from build123d import *

# Parameters (mm, degrees)
F0_W     = 25.4
F0_H     = 25.4
F1_DEPTH = 50.8
F2_W     = 20.32
F2_H     = 45.72
F3_DEPTH = 22.86
F4_R     = 3.175
F4_R_2   = 1.905
F5_DEPTH = 10.16
F6_DEPTH = 25.4
F7_R     = 5.08
F8_DEPTH = 2.54


with BuildPart() as f1:
    # F0 (on Top) → F1 (new body)
    with BuildSketch(Plane.XY):
        with Locations((-10.5220779449, -6.5101005034)):
            Rectangle(F0_W, F0_H)
    extrude(amount=F1_DEPTH)

    # F2 (on face) → F3 (cut)
    with BuildSketch(Plane(origin=(0, 6.1898994966, 0), x_dir=(-1, 0, 0), z_dir=(0, 1, 0))):
        with Locations((10.5220779449, 25.4)):
            Rectangle(F2_W, F2_H)
    extrude(amount=-F3_DEPTH, mode=Mode.SUBTRACT)

    # F4 (on face) → F5 (join)
    with BuildSketch(Plane(origin=(0, -16.6701005034, 0), x_dir=(-1, 0, 0), z_dir=(0, 1, 0))):
        with Locations((11.9491452351, 36.013584584)):
            Circle(F4_R)
        with Locations((11.9491452351, 36.013584584)):
            Circle(F4_R_2, mode=Mode.SUBTRACT)
        with Locations((11.369979009, 16.9800035655)):
            Circle(F4_R)
        with Locations((11.369979009, 16.9800035655)):
            Circle(F4_R_2, mode=Mode.SUBTRACT)
    extrude(amount=F5_DEPTH)

    # F6 (cut): faces of the model
    f6_faces = [f1.faces().sort_by_distance(p)[0] for p in [
        (-11.9491452351, -16.6701005034, 36.013584584),
        (-11.369979009, -16.6701005034, 16.9800035655),
    ]]
    extrude(f6_faces, amount=-F6_DEPTH, mode=Mode.SUBTRACT)

    # F7 (on face) → F8 (join)
    with BuildSketch(Plane(origin=(0, -16.6701005034, 0), x_dir=(-1, 0, 0), z_dir=(0, 1, 0))):
        with Locations((11.369979009, 16.9800035655)):
            Circle(F7_R)
        with Locations((11.9491452351, 36.013584584)):
            Circle(F7_R)
    extrude(amount=F8_DEPTH)


solid = f1.part
Build history of the part. All positions in model axes, mm. A direction names the side the tool comes from. Give positions to 0.01 mm unless a question says otherwise; leave off trailing zeros. Write each loop counter-clockwise with the first axis right and the second up, starting at its lowest first coordinate (ties: lowest second). Pieces come first, ordered by that corner, then holes. Notation, with made-up numbers: (75, -18.75) - (101, -18.75) arc R31 ccw to (101, 15.25) - close; hole circle Ø4 at (33.5, -35.75). An arc over 180 degrees is marked (long way). Use one line per item in the form item = value. Start each with the question number.
1. Band-saw the part on B-B on y = 4. Write the cut outline in (x, z).
2. Band-saw the part on C-C on z = 4. Write the cut outline in (x, y).
3. Band-saw the part on A-A on y = -12. Write the cut outline in (x, z) (3 decimals).
4. Band-saw the part on D-D on x = -18.5. Write the cut outline in (y, z).
5. Drop flat-ended pins along their axis: pin 1 Ø3 at (x, z) = (-11.95, 36.01) entering from +Y; pin 2 Ø8 at (x, z) = (-12, 33.5) entering from +Y; pin 3 Ø5 at (x, z) = (-3.5, 28.5) entering from +Y. Give the stop position or say it passes through.
6. Probe line 1 (Z direction, x = -17.5, y = -13.5); line 2 (X direction, y = -4, z = 32); line 3 (Z direction, x = -12.5, y = -10.5). List the from-to ranges inside material, lowest first. Write a range as [from, to].
7. Two-plate mould, pull along Z, no slides. Class faces 4 (the face through (-23.222, -7, 25)), 5 (the face through (-11, -6, 0)), 6 (the face through (-10, -5, 48.26)): released by +Z, released by -Z, zero draft, split by the parting line, or undercut.
8. 3-axis set-ups, long thin cutter, end or side, ignore diameter. For faces 1 (the face through (-11, -6, 50.8)), 2 (the face through (-12.25, -10.37, 15.29)), 3 (the face through (-12.97, -17.92, 37.62)): which of +Z, -Z, +X, -X, +Y, -Y reach the whole face in a straight line?
Conclusion:
q1.outline = (-23.22, 0) - (2.18, 0) - (2.18, 50.8) - (-23.22, 50.8) - close; hole (-20.68, 2.54) - (-0.36, 2.54) - (-0.36, 48.26) - (-20.68, 48.26) - close
q2.outline = (-23.22, -19.21) - (2.18, -19.21) - (2.18, 6.19) - (-0.36, 6.19) - (-0.36, -16.67) - (-20.68, -16.67) - (-20.68, 6.19) - (-23.22, 6.19) - close
q3.outline = (-23.222, 0) - (2.178, 0) - (2.178, 50.8) - (-23.222, 50.8) - close; circle Ø6.35 at (-11.949, 36.014); circle Ø6.35 at (-11.37, 16.98); hole (-20.682, 2.54) - (-0.362, 2.54) - (-0.362, 48.26) - (-20.682, 48.26) - close; hole circle Ø3.81 at (-11.949, 36.014); hole circle Ø3.81 at (-11.37, 16.98)
q4.outline = (-19.21, 0) - (6.19, 0) - (6.19, 2.54) - (-16.67, 2.54) - (-16.67, 48.26) - (6.19, 48.26) - (6.19, 50.8) - (-19.21, 50.8) - close
q5.pin_1 = -14.13
q5.pin_2 = -6.51
q5.pin_3 = -16.67
q6.line_1 = [0, 2.54], [48.26, 50.8]
q6.line_2 = [-23.22, -20.68], [-0.36, 2.18]
q6.line_3 = [0, 2.54], [14.01, 15.45], [18.51, 19.95], [32.89, 34.19], [37.84, 39.14], [48.26, 50.8]
q7.face_4 = zero draft
q7.face_5 = released by -Z
q7.face_6 = undercut
q8.face_1 = +Z, +X, -X, +Y, -Y
q8.face_2 = +Y
q8.face_3 = -Y
